from build123d import *

# Parameters (mm, degrees)
F1_DEPTH     = 25.4
F2_R         = 7.7705666036
F2_R_2       = 8.2168581005
F3_DEPTH     = 25.4
F4_W         = 43.6024717055
F4_H         = 16.7242367752
F5_DEPTH     = 25.4
F6_R         = 5.2303111982
F7_DEPTH     = 66.548
F8_DEPTH     = 50.546
F9_W         = 14.0256546438
F9_H         = 16.4745816305
F10_DEPTH    = 27.4765354039
F11_T1_DEPTH = 61.3270374103
F11_T3_DEPTH = 60.2313163778


# Not quite as in the source:
# - a fillet or chamfer that OpenCascade refuses, or shapes differently, is made with other operations: its cross-section is extruded or revolved along the edge and cut away or added


with BuildPart() as f1:
    # F0 (on Front) → F1 (new body)
    with BuildSketch(Plane.XZ):
        with BuildLine():
            Line((53.756467998, 21.8012407422), (-22.6971805096, 21.8012407422))
            ThreePointArc((-22.6971805096, 21.8012407422), (-41.5119482204, 2.9864730313), (-22.6971805096, -15.8282946795))
            Line((-22.6971805096, -15.8282946795), (53.756467998, -15.8282946795))
            ThreePointArc((53.756467998, -15.8282946795), (72.5712357089, 2.9864730313), (53.756467998, 21.8012407422))
        make_face()
    extrude(amount=-F1_DEPTH)

    # F2 (on Front) → F3 (cut)
    with BuildSketch(Plane.XZ):
        with Locations((-22.6971805096, 0)):
            Circle(F2_R)
        with Locations((54.9510717392, 0)):
            Circle(F2_R_2)
    extrude(amount=-F3_DEPTH, mode=Mode.SUBTRACT)

    # F4 (on Front) → F5 (join)
    with BuildSketch(Plane.XZ):
        with Locations((15.2310032863, 2.6878237259)):
            Rectangle(F4_W, F4_H)
    extrude(amount=F5_DEPTH)

    # F6 (on Right) → F7 (cut)
    with BuildSketch(Plane.YZ):
        with Locations((-12.524679536, 2.001857613)):
            Circle(F6_R)
    extrude(amount=F7_DEPTH, mode=Mode.SUBTRACT)

    # F6 (on Right) → F8 (cut)
    with BuildSketch(Plane.YZ):
        with Locations((-12.524679536, 2.001857613)):
            Circle(F6_R)
    extrude(amount=-F8_DEPTH, mode=Mode.SUBTRACT)

    # F9 (on face) → F10 (cut, through all)
    with BuildSketch(Plane(origin=(0, 0, -5.6742946617), x_dir=(1, 0, 0), z_dir=(0, 0, -1))):
        with Locations((15.7788638026, 17.1627091847)):
            Rectangle(F9_W, F9_H)
        with BuildLine():
            Line((22.7916911244, 8.9254183695), (8.7660364807, 8.9254183695))
            ThreePointArc((8.7660364807, 8.9254183695), (15.7788638026, 1.9125910476), (22.7916911244, 8.9254183695))
        make_face()
    extrude(amount=-F10_DEPTH, mode=Mode.SUBTRACT)

    # F11: fillet of radius 9.1981536726 on 4 edges, made by hand

    # F11_s2 → F11_t1 (cut)
    with BuildSketch(Plane.YZ.offset(-29.565616748)):
        with BuildLine():
            ThreePointArc((-16.2018463274, -5.6742946617), (-22.7059231637, -2.9802178254), (-25.4, 3.5238590109))
            Line((-25.4, 3.5238590109), (-25.4, -5.6742946617))
            Line((-25.4, -5.6742946617), (-16.2018463274, -5.6742946617))
        make_face()
        with BuildLine():
            ThreePointArc((-16.2018463274, 11.0499421135), (-22.7059231637, 8.3558652771), (-25.4, 1.8517884408))
            Line((-25.4, 1.8517884408), (-25.4, 11.0499421135))
            Line((-25.4, 11.0499421135), (-16.2018463274, 11.0499421135))
        make_face()
    extrude(amount=F11_T1_DEPTH, mode=Mode.SUBTRACT)

    # F11_s4 → F11_t3 (cut)
    with BuildSketch(Plane.YZ.offset(-0.2036930572)):
        with BuildLine():
            ThreePointArc((-16.2018463274, -5.6742946617), (-22.7059231637, -2.9802178254), (-25.4, 3.5238590109))
            Line((-25.4, 3.5238590109), (-25.4, -5.6742946617))
            Line((-25.4, -5.6742946617), (-16.2018463274, -5.6742946617))
        make_face()
        with BuildLine():
            ThreePointArc((-16.2018463274, 11.0499421135), (-22.7059231637, 8.3558652771), (-25.4, 1.8517884408))
            Line((-25.4, 1.8517884408), (-25.4, 11.0499421135))
            Line((-25.4, 11.0499421135), (-16.2018463274, 11.0499421135))
        make_face()
    extrude(amount=F11_T3_DEPTH, mode=Mode.SUBTRACT)


solid = f1.part
Build history of the part. All positions in model axes, mm. A direction names the side the tool comes from. Coordinates: 2 decimals unless noted, no trailing zeros. Order: outer loops, then holes, each group sorted by start corner. A loop starts at its lowest first (then second) coordinate and runs counter-clockwise, first axis right, second up. Notation, with made-up numbers: (77.5, 30.25) - (81.5, 30.25) arc R24 ccw to (81.5, 44.25) - close; hole circle Ø10 at (-0.5, 71). An arc over 180 degrees is marked (long way). Put each result on its own line as item: value.
1. Pull direction Z, two halves, no side cores. Call faces 1 (the face through (-6.57, -7, 3)), 2 (the face through (0.99, -22.33, 8.71)), 3 (the face through (62.788, 12.522, 2.468)): pulls with the +Z half, pulls with the -Z half, needs draft (parallel to the pull), parting line crosses it, or undercut.
Answer sheet:
face 1: needs draft
face 2: pulls with the +Z half
face 3: undercut
2. Probe line 1 along X through (y, z) = (-9, -5); line 2 along X through (y, z) = (10, 2); line 3 along Y through (x, z) = (-24, 15.5). List the from-to ranges inside material, lowest first. Write a range as [from, to].
Answer sheet:
line 1: x = [-6.57, 8.77], [22.79, 37.03]
line 2: x = [-41.49, -30.21], [-15.19, 46.98], [62.92, 72.55]
line 3: y = [0, 25.4]
3. Saw through at C-C (z = 0). Write the cut outline in (x, y), and give its area (3 significant figures).
Answer sheet:
outline: (-41.27, 0) - (-30.47, 0) - (-30.47, 25.4) - (-41.27, 25.4) - close; (-14.93, 0) - (-6.57, 0) - (-6.57, -7.69) - (8.88, -7.69) arc R7.01 cw to (22.68, -7.69) - (37.03, -7.69) - (37.03, 0) - (46.73, 0) - (46.73, 25.4) - (-14.93, 25.4) - close; (-6.57, -24.7) - (8.77, -24.7) - (8.77, -17.36) - (-6.57, -17.36) - close; (22.79, -24.7) - (37.03, -24.7) - (37.03, -17.36) - (22.79, -17.36) - close; (63.17, 0) - (72.33, 0) - (72.33, 25.4) - (63.17, 25.4) - close
area: 2,570 mm^2
4. Saw through at D-D (x = 35). Write the cut outline in (y, z).
Answer sheet:
outline: (-25.36, 2.69) arc R9.2 ccw to (-16.2, -5.67) - (0, -5.67) - (0, -15.83) - (25.4, -15.83) - (25.4, 21.8) - (0, 21.8) - (0, 11.05) - (-16.2, 11.05) arc R9.2 ccw to start; hole circle Ø10.46 at (-12.52, 2)
5. Tool access for faces 4 (the face through (72.567, 12.522, 2.573)), 5 (the face through (22.792, -19, 3)), 6 (the face through (10, -4, -5.674)), 7 (the face through (10, -4, 11.05)): list every direction of +Z, -Z, +X, -X, +Y, -Y with a clear straight run to the whole face (end or side of a thin tool).
Answer sheet:
face 4: +X, +Y, -Y
face 5: +Z, -Z, -Y
face 6: -Z, +X, -X, -Y
face 7: +Z, +X, -X, -Y
6. Saw through at B-B (x = 60). Write the cut outline in (y, z).
Answer sheet:
outline: (0, -14.76) - (25.4, -14.76) - (25.4, -6.48) - (0, -6.48) - close; (0, 6.48) - (25.4, 6.48) - (25.4, 20.74) - (0, 20.74) - close
7. Drop flat-ended pins along their axis: P1, Ø5, axis at y = -11, z = 1, coming from the +X side; P2, Ø8, axis at y = -5, z = 10.5, coming from the -X side; P3, Ø1.5, axis at y = -19.5, z = 9, coming from the +X side; P4, Ø2, axis at y = 14, z = 15, coming from the -X side. Give the stop position or say it passes through.
Answer sheet:
P1: passes through
P2: stops at x = -6.57
P3: stops at x = 37.03
P4: stops at x = -37.95
8. Saw through at A-A (y = 3). Write the cut outline in (x, z), and give its area (3 significant figures).
Answer sheet:
outline: (-22.7, -15.83) - (53.76, -15.83) arc R18.81 ccw to (53.76, 21.8) - (-22.7, 21.8) arc R18.81 ccw to start; hole circle Ø15.54 at (-22.7, 0); hole circle Ø16.43 at (54.95, 0)
area: 3,590 mm^2
